Geometry: final body of the model. Coordinates: model frame, mm. A direction names the side the tool comes from. Give positions to 0.01 mm unless a question says otherwise; leave off trailing zeros. Write each loop counter-clockwise with the first axis right and the second up, starting at its lowest first coordinate (ties: lowest second). Pieces come first, ordered by that corner, then holes. Notation, with made-up numbers: M 6,30.5 L 45,30.5 A36 ccw 45,68.5 Z; hole C 86.25,3 d3. An arc over 180 degrees is marked long. Use a Markdown table: item, result. Add a question column.
(1) Draft query along X for faces 3 (the cylindrical face through (-62.899, 34.948, 0.493)), 4 (the flat face through (-69, 53, -4)), 5 (the cylindrical face through (-59.026, 48.418, -1.824)), 6 (the cylindrical face through (-65.526, 54.918, -1.824)). Return one class per face: released by +X, released by -X, zero draft, split by the parting line, or undercut.
(2) Cut plane B-B (y = 35.25). Output: boundary loops of the cut face in (x, z), plus the area to 3 significant figures.
(3) Reachability of faces 1 (the flat face through (-69, 47, 0)), 2 (the flat face through (-63, 47, -4)) from +Z, -Z, +X, -X, +Y, -Y: full face, straight path, thin tool, end or side. Return the list, or none.
(4) Pin query (flat end, axial travel): pin 1 Ø1 at (y, z) = (40, -3) entering from -X; pin 2 Ø3 at (x, z) = (-61.5, -0.5) entering from -Y; pin 3 Ø3 at (y, z) = (44, -0.5) entering from +X. Return the tip coordinate at first contact, or that it passes through.
(5) Material intervals for L1, parallel to Y at x = -69, z = 0.6; L2, parallel to Z at x = -57.25, y = 41.5; L3, parallel to X at y = 40.5, z = -2.25, sorted ascending.
(6) Cut plane A-A (z = -3.1). Output: boundary loops of the cut face in (x, y), plus the area to 3 significant figures.
```python
from build123d import *

# Parameters (mm, degrees)
F0_R     = 13.5
F1_DEPTH = 1
F2_R     = 3.9
F3_DEPTH = 4
F4_R     = 0.3


with BuildPart() as f1:
    # F0 (on Top) → F1 (new body)
    with BuildSketch(Plane.XY):
        with Locations((-69.12829, 46.924345)):
            Circle(F0_R)
    extrude(amount=F1_DEPTH)

    # F2 (on face) → F3 (join)
    with BuildSketch(Plane(origin=(0, 0, 0), x_dir=(1, 0, 0), z_dir=(0, 0, -1))):
        with Locations((-62.62829, -46.924345)):
            Circle(F2_R)
        with Locations((-69.12829, -40.424345)):
            Circle(F2_R)
        with Locations((-75.62829, -46.924345)):
            Circle(F2_R)
        with Locations((-69.12829, -53.424345)):
            Circle(F2_R)
    extrude(amount=F3_DEPTH)

    # F4
    f4_edges = [f1.edges().sort_by_distance(p)[0] for p in [
        (-73.02829, 53.424345, -4),
        (-66.52829, 46.924345, -4),
        (-73.02829, 40.424345, -4),
        (-79.52829, 46.924345, -4),
    ]]
    fillet(f4_edges, radius=F4_R)


solid = f1.part
```
Answer list:
| question | item | result |
|---|---|---|
| 1 | face 3 | split by the parting line |
| 1 | face 4 | zero draft |
| 1 | face 5 | undercut |
| 1 | face 6 | undercut |
| 2 | outline | M -75.91,0 L -62.35,0 L -62.35,1 L -75.91,1 Z |
| 2 | area | 13.6 mm² |
| 3 | face 1 | -Z |
| 3 | face 2 | -Z, +X, -X, +Y, -Y |
| 4 | pin 1 | x = -73.03 |
| 4 | pin 2 | y = 34.94 |
| 4 | pin 3 | x = -55.71 |
| 5 | L1 | 33.42 to 60.42 |
| 5 | L2 | 0 to 1 |
| 5 | L3 | -73.03 to -65.23 |
| 6 | outline | C -75.63,46.92 d7.8; C -69.13,40.42 d7.8; C -69.13,53.42 d7.8; C -62.63,46.92 d7.8 |
| 6 | area | 191 mm² |
